For this review, use the dimensioned drawing (mm, ordinates from the lowest corner) and the shaded views. A direction names the side the tool comes from. Round coordinates to 2 decimals unless told otherwise and drop trailing zeros. Write each loop counter-clockwise with the first axis right and the second up, starting at its lowest first coordinate (ties: lowest second). Pieces come first, ordered by that corner, then holes.
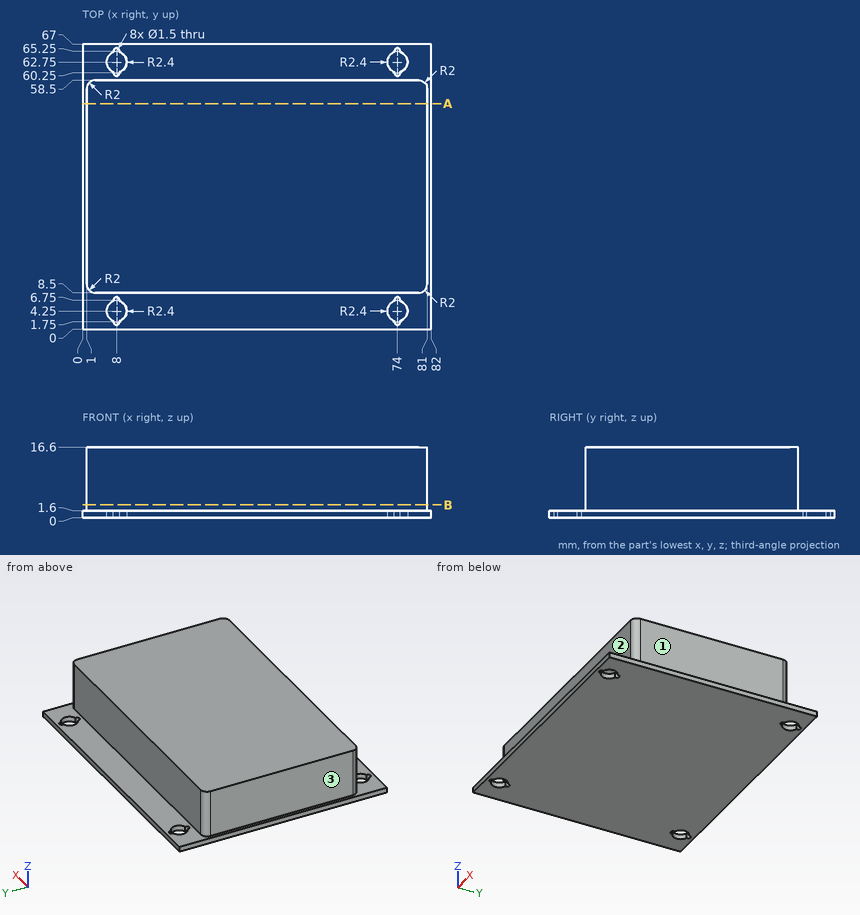
(1) We need section B-B, the plane z = 3. Give the boundary of the cut face in (x, y).
Geometry check:
outline: (1, 10.5) arc R2 ccw to (3, 8.5) - (79, 8.5) arc R2 ccw to (81, 10.5) - (81, 56.5) arc R2 ccw to (79, 58.5) - (3, 58.5) arc R2 ccw to (1, 56.5) - close
(2) For pin 1 Ø0.9 at (x, y) = (8, 60.25) entering from +Z; pin 2 Ø1.7 at (x, y) = (74, 1.75) entering from +Z; pin 3 Ø3 at (x, z) = (32, 8) entering from +Y; pin 4 Ø3 at (y, z) = (51.5, 8) entering from +X, all flat-tipped, find the tip position at first contact; note any pin that passes through.
Geometry check:
pin 1: passes through
pin 2: stops at z = 1.6
pin 3: stops at y = 58.5
pin 4: stops at x = 81
(3) We need section A-A, the plane y = 53. Give the boundary of the cut face in (x, z), and give its area (3 significant figures).
Geometry check:
outline: (0, 0) - (82, 0) - (82, 1.6) - (81, 1.6) - (81, 16.6) - (1, 16.6) - (1, 1.6) - (0, 1.6) - close
area: 1,330 mm2
(4) For line 1 along X through (y, z) = (65.25, 0.8); line 2 along Y through (x, z) = (64.5, 8.75); line 3 along X through (y, z) = (47.5, 3.25), list the stretches that pass through material, from the lowest coordinate up.
Geometry check:
line 1: x = 0 to 7.25, 8.75 to 73.25, 74.75 to 82
line 2: y = 8.5 to 58.5
line 3: x = 1 to 81
(5) For the marked faces 1, 2 and 3, list the 3-axis set-ups (+Z, -Z, +X, -X, +Y, -Y) from which the entire face can be reached by the end or side of a thin tool; tool diameter is ignored.
Geometry check:
face 1: +Z, +X, +Y, -Y
face 2: +Z, +X, -X, -Y
face 3: +Z, -X, +Y, -Y
